Input: part model. Units: mm. Frame: model coordinates. Face numbers are marked on the shaded views. Coordinates: 2 decimals unless noted, no trailing zeros. Write each loop counter-clockwise with the first axis right and the second up, starting at its lowest first coordinate (ties: lowest second). Pieces come first, ordered by that corner, then holes. Notation, with made-up numbers: (-36.5, 40.25) - (-24.5, 40.25) arc R34 ccw to (-24.5, 78.25) - close; hole circle Ø4 at (-32.75, 35.25). An arc over 180 degrees is marked (long way). Use a Markdown table: item, result. Add a question column.
Q1. Section query B-B (x = 135.5). Return the cut outline in (y, z), then the cut area to 3 significant figures.
Q2. Mould query, pull axis X, two halves, no side actions, for the marked faces 1 and 2. Classes: released by +X, released by -X, zero draft, split by the parting line, or undercut.
Q3. Section query A-A (y = -8.25). Return the cut outline in (x, z).
Q4. Pin query (flat end, axial travel): P1, Ø12, axis at x = 72.5, z = 247, coming from the +Y side; P2, Ø2.5, axis at x = 251, y = -8.5, coming from the +Z side; P3, Ø4, axis at x = 18.07, z = -39.71, coming from the -Y side; P4, Ø1.1, axis at x = -35, y = -3.5, coming from the -Z side. Return the tip coordinate at first contact, or that it passes through.
Q5. Material intervals for probe 1 along X at (y, z) = (-10.25, 284); probe 2 along X at (y, z) = (-1.75, 235); probe 3 along Y at (x, z) = (142, 91), sorted ascending. Write a range as from..to.
Q6. Section query D-D (z = 30.5). Return the cut outline in (x, y).
Q7. Section query C-C (z = 183.5). Return the cut outline in (x, y), then the cut area to 3 significant figures.
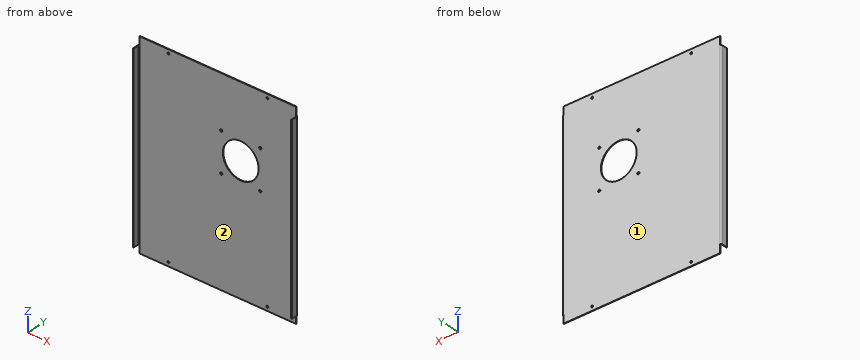
from build123d import *

# Parameters (mm, degrees)
SKETCH_1_W                         = 287
SKETCH_1_H                         = 358
SM_BASE_FLANGE_1_DEPTH             = 1
SM_EDGE_FLANGE_1_STRIP_W           = 6.2
SM_EDGE_FLANGE_1_STRIP_H           = 1
SM_EDGE_FLANGE_1_STRIP_CUT_DEPTH   = 358
SM_EDGE_FLANGE_1_STRIP_2_W         = 6.2
SM_EDGE_FLANGE_1_STRIP_2_H         = 1
SM_EDGE_FLANGE_1_STRIP_CUT_2_DEPTH = 358
SM_EDGE_FLANGE_1_DEPTH             = 358
SM_EDGE_FLANGE_1_BEND_DEPTH        = 358
SKETCH_10_W                        = 15
SKETCH_10_H                        = 15
CUT_EXTRUDE_2_DEPTH                = 2.1
SKETCH_11_W                        = 15
SKETCH_11_H                        = 14.697316693
CUT_EXTRUDE_3_DEPTH                = 2.1
SKETCH_12_W                        = 15
SKETCH_12_H                        = 14.830573141
CUT_EXTRUDE_4_DEPTH                = 2.1
SKETCH_13_W                        = 15
SKETCH_13_H                        = 16.610777732
CUT_EXTRUDE_5_DEPTH                = 2.1
SKETCH_14_R                        = 1.75
CUT_EXTRUDE_6_DEPTH                = 10
SKETCH_15_R                        = 32.5
CUT_EXTRUDE_7_DEPTH                = 10
SKETCH_16_R                        = 2
CUT_EXTRUDE_8_DEPTH                = 10


# Sheet-metal steps are written as plain solids
with BuildPart() as part:
    # Sketch 1 → Базовая кромка1 (new body)
    with BuildSketch(Plane(origin=(0, 0, 0), x_dir=(1, 0, 0), z_dir=(0, 1, 0))):
        with Locations((108.072246785, -132.29374857)):
            Rectangle(SKETCH_1_W, SKETCH_1_H)
    extrude(amount=-SM_BASE_FLANGE_1_DEPTH)

    # Ребро-кромка1 strip (across the edge) → Ребро-кромка1 strip cut (cut)
    with BuildSketch(Plane(origin=(251.572246785, -1, -46.70625143), x_dir=(-1, 0, 0), z_dir=(0, 0, 1))):
        with Locations((-2, -0.5)):
            Rectangle(SM_EDGE_FLANGE_1_STRIP_W, SM_EDGE_FLANGE_1_STRIP_H)
    extrude(amount=SM_EDGE_FLANGE_1_STRIP_CUT_DEPTH, mode=Mode.SUBTRACT)

    # Ребро-кромка1 strip 2 (across the edge) → Ребро-кромка1 strip cut 2 (cut)
    with BuildSketch(Plane(origin=(-35.427753215, -1, 311.29374857), x_dir=(1, 0, 0), z_dir=(0, 0, -1))):
        with Locations((-2, -0.5)):
            Rectangle(SM_EDGE_FLANGE_1_STRIP_2_W, SM_EDGE_FLANGE_1_STRIP_2_H)
    extrude(amount=SM_EDGE_FLANGE_1_STRIP_CUT_2_DEPTH, mode=Mode.SUBTRACT)

    # Ребро-кромка1 section (across the edge) → Ребро-кромка1 (add)
    with BuildSketch(Plane(origin=(251.572246785, -1, -46.70625143), x_dir=(-1, 0, 0), z_dir=(0, 0, 1))):
        with BuildLine():
            Line((-1, 1.1), (-1, 12))
            Line((-1, 12), (0, 12))
            Line((0, 12), (0, 1.1))
            ThreePointArc((0, 1.1), (0.322182541, 0.322182541), (1.1, 0))
            Line((1.1, 0), (1.1, -1))
            ThreePointArc((1.1, -1), (-0.38492424, -0.38492424), (-1, 1.1))
        make_face()
    extrude(amount=SM_EDGE_FLANGE_1_DEPTH)

    # Ребро-кромка1 section 2 (across the edge) → Ребро-кромка1 bend (add)
    with BuildSketch(Plane(origin=(-35.427753215, -1, 311.29374857), x_dir=(1, 0, 0), z_dir=(0, 0, -1))):
        with BuildLine():
            Line((-1, 1.1), (-1, 12))
            Line((-1, 12), (0, 12))
            Line((0, 12), (0, 1.1))
            ThreePointArc((0, 1.1), (0.322182541, 0.322182541), (1.1, 0))
            Line((1.1, 0), (1.1, -1))
            ThreePointArc((1.1, -1), (-0.38492424, -0.38492424), (-1, 1.1))
        make_face()
    extrude(amount=SM_EDGE_FLANGE_1_BEND_DEPTH)

    # Эскиз10 → Вырез-Вытянуть2 (cut)
    with BuildSketch(Plane(origin=(252.572246785, 0, 0), x_dir=(0, 0, -1), z_dir=(1, 0, 0))):
        with Locations((39.20625143, -5.5)):
            Rectangle(SKETCH_10_W, SKETCH_10_H)
    extrude(amount=-CUT_EXTRUDE_2_DEPTH, mode=Mode.SUBTRACT)

    # Эскиз11 → Вырез-Вытянуть3 (cut)
    with BuildSketch(Plane(origin=(252.572246785, 0, 0), x_dir=(0, 0, -1), z_dir=(1, 0, 0))):
        with Locations((-303.79374857, -5.651341654)):
            Rectangle(SKETCH_11_W, SKETCH_11_H)
    extrude(amount=-CUT_EXTRUDE_3_DEPTH, mode=Mode.SUBTRACT)

    # Эскиз12 → Вырез-Вытянуть4 (cut)
    with BuildSketch(Plane.ZY.offset(36.427753215)):
        with Locations((303.79374857, -5.584713429)):
            Rectangle(SKETCH_12_W, SKETCH_12_H)
    extrude(amount=-CUT_EXTRUDE_4_DEPTH, mode=Mode.SUBTRACT)

    # Эскиз13 → Вырез-Вытянуть5 (cut)
    with BuildSketch(Plane.ZY.offset(36.427753215)):
        with Locations((-39.20625143, -4.694611134)):
            Rectangle(SKETCH_13_W, SKETCH_13_H)
    extrude(amount=-CUT_EXTRUDE_5_DEPTH, mode=Mode.SUBTRACT)

    # Эскиз14 → Вырез-Вытянуть6 (cut)
    with BuildSketch(Plane(origin=(0, 0, 0), x_dir=(1, 0, 0), z_dir=(0, 1, 0))):
        with Locations(Location((18.072246785, -304.29374857, 0), (0, 0, 270))):
            Circle(SKETCH_14_R)
        with Locations(Location((198.072246785, -304.29374857, 0), (0, 0, 270))):
            Circle(SKETCH_14_R)
        with Locations(Location((18.072246785, 39.70625143, 0), (0, 0, 270))):
            Circle(SKETCH_14_R)
        with Locations(Location((198.072246785, 39.70625143, 0), (0, 0, 270))):
            Circle(SKETCH_14_R)
    extrude(amount=-CUT_EXTRUDE_6_DEPTH, mode=Mode.SUBTRACT)

    # Эскиз15 → Вырез-Вытянуть7 (cut)
    with BuildSketch(Plane(origin=(0, 0, 0), x_dir=(1, 0, 0), z_dir=(0, 1, 0))):
        with Locations(Location((149.710381915, -181.167811182, 0), (0, 0, 270))):
            Circle(SKETCH_15_R)
    extrude(amount=-CUT_EXTRUDE_7_DEPTH, mode=Mode.SUBTRACT)

    # Эскиз16 → Вырез-Вытянуть8 (cut)
    with BuildSketch(Plane.XZ.offset(1)):
        with Locations(Location((114.21015579, 216.667585055, 0), (0, 0, 270))):
            Circle(SKETCH_16_R)
        with Locations(Location((185.210155788, 216.668037307, 0), (0, 0, 270))):
            Circle(SKETCH_16_R)
        with Locations(Location((114.210608042, 145.667585057, 0), (0, 0, 270))):
            Circle(SKETCH_16_R)
        with Locations(Location((185.21060804, 145.668037309, 0), (0, 0, 270))):
            Circle(SKETCH_16_R)
    extrude(amount=-CUT_EXTRUDE_8_DEPTH, mode=Mode.SUBTRACT)


solid = part.part
Values follow:
| question | item | result |
|---|---|---|
| 1 | outline | (-1, -46.71) - (0, -46.71) - (0, 151.94) - (-1, 151.94) - close; (-1, 210.4) - (0, 210.4) - (0, 311.29) - (-1, 311.29) - close |
| 1 | area | 300 mm2 |
| 2 | face 1 | zero draft |
| 2 | face 2 | undercut |
| 3 | outline | (-36.43, -31.71) - (-35.43, -31.71) - (-35.43, 296.29) - (-36.43, 296.29) - close; (251.57, -31.71) - (252.57, -31.71) - (252.57, 296.29) - (251.57, 296.29) - close |
| 4 | P1 | y = 0 |
| 4 | P2 | z = 296.29 |
| 4 | P3 | y = -1 |
| 4 | P4 | z = -31.71 |
| 5 | probe 1 | -36.43..-35.43, 251.57..252.57 |
| 5 | probe 2 | -36.4..-35.37, 251.52..252.54 |
| 5 | probe 3 | -1..0 |
| 6 | outline | (-36.43, -13) - (-35.43, -13) - (-35.43, -2.1) arc R1.1 cw to (-34.33, -1) - (250.47, -1) arc R1.1 cw to (251.57, -2.1) - (251.57, -13) - (252.57, -13) - (252.57, -2.1) arc R2.1 ccw to (250.47, 0) - (-34.33, 0) arc R2.1 ccw to (-36.43, -2.1) - close |
| 7 | outline | (-36.43, -13) - (-35.43, -13) - (-35.43, -2.1) arc R1.1 cw to (-34.33, -1) - (117.29, -1) - (117.29, 0) - (-34.33, 0) arc R2.1 ccw to (-36.43, -2.1) - close; (182.13, -1) - (250.47, -1) arc R1.1 cw to (251.57, -2.1) - (251.57, -13) - (252.57, -13) - (252.57, -2.1) arc R2.1 ccw to (250.47, 0) - (182.13, 0) - close |
| 7 | area | 247 mm2 |
